Autodesk Fusion 360 part; units mm, degrees
sketch "Sketch1" plane through (0, 0, 0) normal (0, 0, 1) x (1, 0, 0)
  line L0 (7.5, 0) -> (132.5, 0)
  line L1 (140, 7.5) -> (140, 132.5)
  line L2 (132.5, 140) -> (7.5, 140)
  line L3 (0, 132.5) -> (0, 7.5)
  circle A0 centre (7.5, 132.5) radius 7.5
  circle A1 centre (7.5, 132.5) radius 3
  line L4 (0, 70) -> (140, 70) construction
  line L5 (70, 140) -> (70, 0) construction
  circle A2 centre (7.5, 7.5) radius 3
  circle A3 centre (7.5, 7.5) radius 7.5
  circle A4 centre (132.5, 132.5) radius 7.5
  circle A5 centre (132.5, 132.5) radius 3
  circle A6 centre (132.5, 7.5) radius 3
  circle A7 centre (132.5, 7.5) radius 7.5
  line L6 (7.5, 7.5) -> (132.5, 7.5)
  line L7 (132.5, 7.5) -> (132.5, 132.5)
  line L8 (132.5, 132.5) -> (7.5, 132.5)
  line L9 (7.5, 132.5) -> (7.5, 7.5)
  line L10 (7.5, 92.5) -> (25.5, 92.5)
  line L11 (25.5, 92.5) -> (25.5, 47.5)
  line L12 (25.5, 47.5) -> (7.5, 47.5)
  line L13 (7.5, 47.5) -> (7.5, 92.5)
  line L14 (7.5, 70) -> (25.5, 70) construction
  line L15 (7.5, 94.5) -> (27.5, 94.5)
  line L16 (27.5, 94.5) -> (27.5, 45.5)
  line L17 (27.5, 45.5) -> (7.5, 45.5)
  line L18 (7.5, 45.5) -> (7.5, 94.5)
  line L19 (7.5, 70) -> (27.5, 70) construction
  line L20 (27.5, 132.5) -> (43.5, 132.5)
  line L21 (43.5, 132.5) -> (43.5, 119.9)
  line L22 (43.5, 119.9) -> (27.5, 119.9)
  line L23 (27.5, 119.9) -> (27.5, 132.5)
  line L24 (25.5, 132.5) -> (45.5, 132.5)
  line L25 (45.5, 132.5) -> (45.5, 117.9)
  line L26 (45.5, 117.9) -> (25.5, 117.9)
  line L27 (25.5, 117.9) -> (25.5, 132.5)
  line L28 (35.5, 119.9) -> (35.5, 122) construction
  line L29 (35.5, 117.9) -> (35.5, 122) construction
  dimension "d3" = 15
  dimension "d4" = 6
  dimension "d6" = 140
  dimension "d7" = 140
  dimension "d10" = 45
  dimension "d11" = 18
  dimension "d12" = 49
  dimension "d13" = 20
  dimension "d14" = 16
  dimension "d15" = 12.6
  dimension "d16" = 20
  dimension "d17" = 20
  dimension "d18" = 14.6
extrude "Extrude1" add sketch "Sketch1" along normal blind 10 contours A2 A3 L6 L9 | A6 A7 L6 L7 | A2 A3 L6 L9 | A6 A7 L6 L7 | A0 A1 L8 L9 | A4 A5 L7 L8 | A0 A1 L8 L9 | A4 A5 L7 L8 makes body 1 at (14.9627, 8.2468, 3.3333) makes body 2 at (139.9627, 8.2468, 6.6667) makes body 3 at (14.8513, 133.9861, 6.6667) makes body 4 at (139.4111, 135.4133, 6.6667)
extrude "Extrude1'" add sketch "Sketch1" along normal blind 3 separate body contours L0 A3 A7 L6 | A2 A3 L6 L9 | A6 A7 L6 L7 | L3 A0 A3 L9 L13 L18 | A2 A3 L6 L9 | L1 A4 A7 L7 | A6 A7 L6 L7 | A0 A1 L8 L9 | A4 A5 L7 L8 | L2 A0 A4 L8 L20 L24 | A0 A1 L8 L9 | L9 L10 L11 L12 L15 L16 L17 L18 | A4 A5 L7 L8 | L8 L21 L22 L23 L24 L25 L26 L27 makes body 5 in component "Component"
combine "Combine1" operation add target body 4 tool bodies 5
combine "Combine2" operation add target body 2 tool bodies 4
combine "Combine3" operation add target body 1 tool bodies 2
combine "Combine4" operation add target body 3 tool bodies 1
component "Component" placed x (1, 0, 0) y (0, 1, 0) z (0, 0, 1) at (0, 0, 0)
equation "d2 = d1"
equation "d18 = d15 + 2 mm"
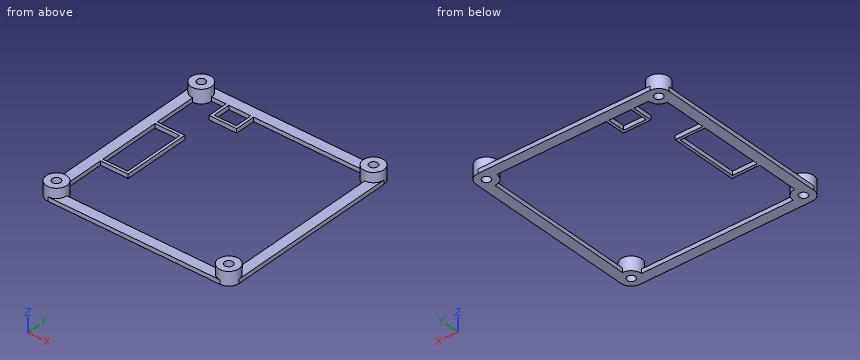
Here's how the part is built. I have some questions about the finished solid (model axes, mm). Coordinates: 2 decimals unless noted, no trailing zeros. Loops run counter-clockwise (first coordinate to the right, second up) from the corner with the lowest first, then second, coordinate; pieces in that order, holes last. Notation, with made-up numbers: (89, 66.5) - (126, 66.5) arc R25 cw to (126, 102.5) - close; hole circle Ø5 at (-10.5, -27). An arc over 180 degrees is marked (long way). Return JSON: item names as keys, results as strings. Group by question number.
Item 1: If we section it at C-C on x = 115.5: Write out the boundary of the cut face in (y, z).
Item 2: If we section it at A-A on z = 6.75: Write out the boundary of the cut face in (x, y), and give its area (3 significant figures).
Item 3: I need wall thicknesses on line 1 (Y direction, x = 7.5, z = 5.25); line 2 (Y direction, x = 100, z = 2.75). Which ranges of each line are inside material? Lowest first, please. Write a range as from..to.
Item 4: If we section it at B-B on y = 64.5: Write out the boundary of the cut face in (x, z), and give its area (3 significant figures).
Item 5: Will this pin go through, and if not, where does the flat tip stop? P1, Ø4, axis at x = 63.5, y = 3, coming from the +Z side.
Calculated:
{
 "1": {"outline": "(0, 0) - (7.5, 0) - (7.5, 3) - (0, 3) - close; (132.5, 0) - (140, 0) - (140, 3) - (132.5, 3) - close"},
 "2": {"outline": "circle Ø15 at (7.5, 7.5); circle Ø15 at (7.5, 132.5); circle Ø15 at (132.5, 7.5); circle Ø15 at (132.5, 132.5); hole circle Ø6 at (7.5, 7.5); hole circle Ø6 at (7.5, 132.5); hole circle Ø6 at (132.5, 7.5); hole circle Ø6 at (132.5, 132.5)", "area": "594 mm^2"},
 "3": {"line 1": "y = 0..4.5, 10.5..15, 125..129.5, 135.5..140", "line 2": "y = 0..7.5, 132.5..140"},
 "4": {"outline": "(0, 0) - (7.5, 0) - (7.5, 3) - (0, 3) - close; (25.5, 0) - (27.5, 0) - (27.5, 3) - (25.5, 3) - close; (132.5, 0) - (140, 0) - (140, 3) - (132.5, 3) - close", "area": "51.0 mm^2"},
 "5": {"P1": "stops at z = 3"}
}
